from build123d import *

# Parameters (mm, degrees)
EXTRUDE_1_DEPTH         = 30
CUT_EXTRUDE_1_DEPTH     = 28
EXTRUDE_START           = 21.5
EXTRUDE_2_DEPTH         = 21.5
CUT_EXTRUDE_2_DEPTH     = 1.5
HOLE_WIZARD_2_2_2_2_1_D = 2.2
CUT_EXTRUDE_3_REACH     = 48.867
SKETCH_7_W              = 25
SKETCH_7_H              = 15
CUT_EXTRUDE_4_REACH     = 66.135
SKETCH_8_W              = 10
SKETCH_8_H              = 5


with BuildPart() as part:
    # 草图1 → 凸台-拉伸1 (new body)
    with BuildSketch(Plane(origin=(0, 0, 0), x_dir=(1, 0, 0), z_dir=(0, 1, 0))):
        with BuildLine():
            Line((-26.5, -24.5), (26.5, -24.5))
            ThreePointArc((26.5, -24.5), (27.914213562, -23.914213562), (28.5, -22.5))
            Line((28.5, -22.5), (28.5, 22.5))
            ThreePointArc((28.5, 22.5), (27.914213562, 23.914213562), (26.5, 24.5))
            Line((26.5, 24.5), (-26.5, 24.5))
            ThreePointArc((-26.5, 24.5), (-27.914213562, 23.914213562), (-28.5, 22.5))
            Line((-28.5, 22.5), (-28.5, -22.5))
            ThreePointArc((-28.5, -22.5), (-27.914213562, -23.914213562), (-26.5, -24.5))
        make_face()
    extrude(amount=EXTRUDE_1_DEPTH)

    # 草图2 → 切除-拉伸1 (cut)
    with BuildSketch(Plane(origin=(0, 30, 0), x_dir=(1, 0, 0), z_dir=(0, 1, 0))):
        with BuildLine():
            Line((-26.5, -23), (26.5, -23))
            ThreePointArc((26.5, -23), (26.853553391, -22.853553391), (27, -22.5))
            Line((27, -22.5), (27, 22.5))
            ThreePointArc((27, 22.5), (26.853553391, 22.853553391), (26.5, 23))
            Line((26.5, 23), (-26.5, 23))
            ThreePointArc((-26.5, 23), (-26.853553391, 22.853553391), (-27, 22.5))
            Line((-27, 22.5), (-27, -22.5))
            ThreePointArc((-27, -22.5), (-26.853553391, -22.853553391), (-26.5, -23))
        make_face()
    extrude(amount=-CUT_EXTRUDE_1_DEPTH, mode=Mode.SUBTRACT)

    # 草图3 → 凸台-拉伸2 (add)
    with BuildSketch(Plane(origin=(0, 2, 0), x_dir=(1, 0, 0), z_dir=(0, 1, 0)).offset(EXTRUDE_START)):
        with BuildLine():
            Line((-27, -16), (-23, -16))
            ThreePointArc((-23, -16), (-20.878679656, -16.878679656), (-20, -19))
            Line((-20, -19), (-20, -23))
            Line((-20, -23), (-26.5, -23))
            ThreePointArc((-26.5, -23), (-26.853553391, -22.853553391), (-27, -22.5))
            Line((-27, -22.5), (-27, -16))
        make_face()
        with BuildLine():
            Line((-27, 16), (-23, 16))
            ThreePointArc((-23, 16), (-20.878679656, 16.878679656), (-20, 19))
            Line((-20, 19), (-20, 23))
            Line((-20, 23), (-26.5, 23))
            ThreePointArc((-26.5, 23), (-26.853553391, 22.853553391), (-27, 22.5))
            Line((-27, 22.5), (-27, 16))
        make_face()
        with BuildLine():
            Line((20, 23), (20, 19))
            ThreePointArc((20, 19), (20.878679656, 16.878679656), (23, 16))
            Line((23, 16), (27, 16))
            Line((27, 16), (27, 22.5))
            ThreePointArc((27, 22.5), (26.853553391, 22.853553391), (26.5, 23))
            Line((26.5, 23), (20, 23))
        make_face()
    extrude(amount=-EXTRUDE_2_DEPTH)

    # 草图4 → 切除-拉伸2 (cut)
    with BuildSketch(Plane.XY.offset(24.5)):
        Polygon((-21.5, 30), (9.5, 30), (9.5, 25), (-8.5, 25), (-8.5, 24), (-21.5, 24), align=None)
    extrude(amount=-CUT_EXTRUDE_2_DEPTH, mode=Mode.SUBTRACT)

    # Ø2.2 (2.2) 直径孔1 (through all)
    with Locations(Plane(origin=(0, 0, 0), x_dir=(-1, 0, 0), z_dir=(0, -1, 0))):
        with Locations((23, -9), (23, 9), (-23, -9), (-23, 9)):
            Hole(HOLE_WIZARD_2_2_2_2_1_D / 2)

    # 草图7 → 切除-拉伸3 (cut, up to next)
    with BuildSketch(Plane(origin=(0, 2, 0), x_dir=(1, 0, 0), z_dir=(0, 1, 0)), mode=Mode.PRIVATE) as cut_extrude_3_sk1:
        Rectangle(SKETCH_7_W, SKETCH_7_H)
    cut_extrude_3_tool1 = extrude(cut_extrude_3_sk1.sketch, amount=-CUT_EXTRUDE_3_REACH, mode=Mode.PRIVATE) & part.part
    add(cut_extrude_3_tool1.solids().sort_by_distance((0, 2, 0))[0], mode=Mode.SUBTRACT)

    # 草图8 → 切除-拉伸4 (cut, up to next)
    with BuildSketch(Plane.XY.offset(24.5), mode=Mode.PRIVATE) as cut_extrude_4_sk1:
        with Locations((0, 15)):
            Rectangle(SKETCH_8_W, SKETCH_8_H)
    cut_extrude_4_tool1 = extrude(cut_extrude_4_sk1.sketch, amount=-CUT_EXTRUDE_4_REACH, mode=Mode.PRIVATE) & part.part
    add(cut_extrude_4_tool1.solids().sort_by_distance((0, 15, 24.5))[0], mode=Mode.SUBTRACT)


solid = part.part
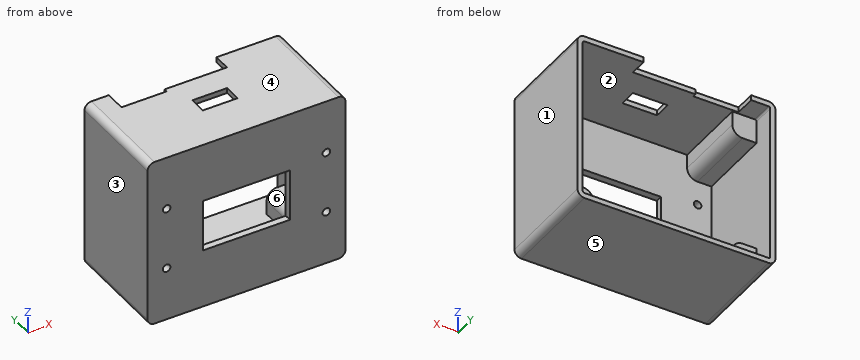
Input: part model. Units: mm. Frame: model coordinates. Face numbers are marked on the shaded views. A direction names the side the tool comes from. Give positions to 0.01 mm unless a question says otherwise; leave off trailing zeros. Write each loop counter-clockwise with the first axis right and the second up, starting at its lowest first coordinate (ties: lowest second). Pieces come first, ordered by that corner, then holes. Notation, with made-up numbers: M 65,23.25 L 116,23.25 A9 cw 116,29.25 Z; hole C -37.75,3 d3. An arc over 180 degrees is marked long. Write item = value, one per line. Start each with the question number.
1) Cut plane D-D on z = 3. Return the cut outline in (x, y).
2) First-contact query: pin 1 Ø1.2 at (y, z) = (14.5, 23.5) entering from +X; pin 2 Ø1.6 at (y, z) = (15.5, 23.5) entering from -X; pin 3 Ø0.8 at (x, z) = (-15.5, 23.5) entering from +Y. Flat tips, straight axial feed; report the tip coordinate or a pass-through.
3) Material intervals for line 1 along Z through (x, y) = (23, 1.4); line 2 along Z through (x, y) = (-4, 1.75); line 3 along Z through (x, y) = (-26, 26.25), sorted ascending. Write a range as [from, to].
4) Draft query along X for the marked faces 1, 2, 3 and 4. Return one class per face: +X half, -X half, draft (parallel to the pull), parting line (faces both ways), or undercut.
5) Cut plane A-A on z = 9. Return the cut outline in (x, y), then the cut area to 3 significant figures.
6) Cut plane B-B on x = 6.5. Return the cut outline in (y, z), then the cut area to 4 significant figures.
7) Cut plane C-C on y = 11.5. Return the cut outline in (x, z).
8) Reachability of the marked faces 5 and 6 from +Z, -Z, +X, -X, +Y, -Y: full face, straight path, thin tool, end or side. Return the list, or none.
Solved:
q1.outline = M -28.5,0 L -12.5,0 L -12.5,2 L -27,2 L -27,30 L -28.5,30 Z; M 12.5,0 L 28.5,0 L 28.5,30 L 27,30 L 27,2 L 12.5,2 Z
q2.pin_1 = 28.46
q2.pin_2 = -28.49
q2.pin_3 = 24
q3.line_1 = [-24.5, -10.1], [-7.9, 7.9], [10.1, 24.5]
q3.line_2 = [-24.5, -7.5], [7.5, 24.5]
q3.line_3 = [-24.5, -23], [23, 24.5]
q4.face_1 = +X half
q4.face_2 = undercut
q4.face_3 = -X half
q4.face_4 = draft
q5.outline = M -28.5,0 L -24.1,0 L -24.1,2 L -27,2 L -27,30 L -28.5,30 Z; M -21.9,0 L 21.9,0 L 21.9,2 L -21.9,2 Z; M 24.1,0 L 28.5,0 L 28.5,30 L 27,30 L 27,2 L 24.1,2 Z
q5.area = 189 mm2
q6.outline = M 0,-24.5 L 30,-24.5 L 30,-23 L 2,-23 L 2,-7.5 L 0,-7.5 Z; M 0,7.5 L 2,7.5 L 2,23 L 25,23 L 25,24.5 L 0,24.5 Z
q6.area = 144.5 mm2
q7.outline = M -28.5,-22.5 A2 ccw -26.5,-24.5 L 26.5,-24.5 A2 ccw 28.5,-22.5 L 28.5,22.5 A2 ccw 26.5,24.5 L -26.5,24.5 A2 ccw -28.5,22.5 Z; hole M -27,-16 L -23,-16 A3 cw -20,-19 L -20,-23 L 20,-23 L 20,-19 A3 cw 23,-16 L 27,-16 L 27,22.5 A0.5 ccw 26.5,23 L -20,23 L -20,19 A3 cw -23,16 L -27,16 Z
q8.face_5 = -Z, +X, -X, +Y, -Y
q8.face_6 = +Y
